The listing builds one solid part. Answer for the finished solid, in the listing's coordinates (mm). A direction names the side the tool comes from. Round coordinates to 2 decimals unless told otherwise and drop trailing zeros. Loops run counter-clockwise (first coordinate to the right, second up) from the corner with the lowest first, then second, coordinate; pieces in that order, holes last. Notation, with made-up numbers: (-19, -4.5) -> (4, -4.5) arc R12 ccw to (4, 2.5) -> close; hole circle Ø2 at (-19.75, 9). An arc over 180 degrees is marked (long way). Write each question's results on one line, items separated by ' | '. Start each with the question number.
(1) Determine the mould class of faces 1 (the face through (10, -8, -3)), 2 (the face through (4.93, 3.377, 3.849)), 3 (the face through (1.6, -11.8, -4)) for opening direction Z: released by +Z, released by -Z, zero draft, split by the parting line, or undercut.
(2) The part is cut by section C-C (y = 0). Determine the outline of the cut face in (x, z), plus the area to 3 significant figures.
(3) Flat-ended cylindrical pins translate along their axes: pin 1 (4 mm diameter, centred on x = 3.5, y = -4, fed in from +Z); pin 2 (2 mm diameter, centred on x = 0.5, z = -0.5, fed in from +Y); pin 3 (1.6 mm diameter, centred on x = 8.5, y = -12.5, fed in from +Z); pin 4 (6.5 mm diameter, centred on y = 0, z = 0, fed in from +X). Find the tip coordinate at first contact, or state that the pin passes through.
(4) The part is cut by section A-A (y = -10.75). Determine the outline of the cut face in (x, z), plus the area to 3 significant figures.
(5) Straight lines are drawn through the part: probe 1 along Z at (x, y) = (7.5, 0); probe 2 along X at (y, z) = (-9.75, 2); probe 3 along Z at (x, y) = (8.25, -17). For each, find the intervals that lie inside material, in ascending order.
(6) For faces 4 (the face through (8, -12, 2)), 5 (the face through (9, -11, -1.5)), 6 (the face through (1.6, -11.6, 4)), determine the directions among +Z, -Z, +X, -X, +Y, -Y from which every point of the face is accessible in a straight line to the end or side of a thin tool.
(7) The part is cut by section D-D (x = 4). Determine the outline of the cut face in (y, z).
(8) The part is cut by section B-B (z = 0). Determine the outline of the cut face in (x, y).
Autodesk Inventor part; units mm, degrees
ref_plane "YZ Plane" through (0, 0, 0) normal (1, 0, 0) x (0, 1, 0)
ref_plane "XZ Plane" through (0, 0, 0) normal (0, 1, 0) x (-1, 0, 0)
ref_plane "XY Plane" through (0, 0, 0) normal (0, 0, 1) x (1, 0, 0)
sketch "Sketch1" plane through (0, 0, 0) normal (1, 0, 0) x (0, 1, 0)
  arc A0 (2, 3.4641) -> (2, -3.4641) centre (0, 0) ccw
  arc A1 (2, 3.4641) -> (3, 5.1962) centre (2.5, 4.3301) ccw
  arc A2 (3, -5.1962) -> (2, -3.4641) centre (2.5, -4.3301) ccw
  line L0 (-4.4721, 4) -> (-19, 4)
  line L1 (-19, 4) -> (-19, -4)
  line L2 (-19, -4) -> (-4.4721, -4)
  arc A3 (3, 5.1962) -> (-4.4721, 4) centre (0, 0) ccw
  arc A4 (-4.4721, -4) -> (3, -5.1962) centre (0, 0) ccw
  point P0 (-6, 0)
  point P1 (-19, 0)
  dimension "d0" = 8
  dimension "d2" = 2.5
  dimension "d3" = 8
  dimension "d6" = 19
  dimension "d7" = 6
  dimension "d8" = 6
extrude "Extrusion1" add sketch "Sketch1" along normal blind 10
sketch "Sketch2" plane through (0, -19, 4) normal (0, 0, 1) x (1, 0, 0)
  line L0 (2, 12) -> (8, 12)
  line L1 (8, 12) -> (8, 2)
  line L2 (8, 2) -> (2, 2)
  line L3 (2, 2) -> (2, 12)
  line L4 (0, 0) -> (10, 0)
  line L5 (10, 14.5279) -> (10, 0)
  point P0 (0, 19)
  dimension "d11" = 2
  dimension "d12" = 6
  dimension "d13" = 10
  dimension "d14" = 2
extrude "Extrusion2" cut sketch "Sketch2" against normal blind 10
sketch "Sketch3" plane through (0, 0, 0) normal (-1, 0, 0) x (0, 0, 1)
  line L0 (-1.5, -7) -> (1.5, -7)
  line L1 (1.5, -7) -> (1.5, -15)
  line L2 (1.5, -15) -> (-1.5, -15)
  line L3 (-1.5, -15) -> (-1.5, -7)
  line L4 (4, -7) -> (-4, -7)
  line L5 (4, -17) -> (-4, -17)
  line L6 (4, -4.4721) -> (4, -19)
  point P0 (0, 0)
  point P1 (0, -7)
  point P2 (0, -7)
  dimension "d17" = 3
  dimension "d18" = 2
  dimension "d19" = 2.5
extrude "Extrusion3" cut sketch "Sketch3" against normal blind 10
properties part number "Thread_Clip"
Checked values:
1) face 1: zero draft | face 2: undercut | face 3: released by -Z
2) outline: (0, -6) -> (10, -6) -> (10, -4) -> (0, -4) -> close; (0, 4) -> (10, 4) -> (10, 6) -> (0, 6) -> close | area: 40.0 mm2
3) pin 1: stops at z = 5.66 | pin 2: stops at y = -3.71 | pin 3: stops at z = 4 | pin 4: passes through
4) outline: (0, -4) -> (2, -4) -> (2, -1.5) -> (0, -1.5) -> close; (0, 1.5) -> (2, 1.5) -> (2, 4) -> (0, 4) -> close; (8, -4) -> (10, -4) -> (10, -1.5) -> (8, -1.5) -> close; (8, 1.5) -> (10, 1.5) -> (10, 4) -> (8, 4) -> close | area: 20.0 mm2
5) probe 1: z = -6 to -4, 4 to 6 | probe 2: x = 0 to 2, 8 to 10 | probe 3: z = -4 to 4
6) face 4: +Z, -Z | face 5: +X, -X | face 6: +Z, +X, -X, -Y
7) outline: (-19, -4) -> (-17, -4) -> (-17, 4) -> (-19, 4) -> close; (-7, -4) -> (-4.47, -4) arc R6 ccw to (3, -5.2) arc R1 ccw to (2, -3.46) arc R4 cw (long way) to (2, 3.46) arc R1 ccw to (3, 5.2) arc R6 ccw to (-4.47, 4) -> (-7, 4) -> close
8) outline: (0, -19) -> (10, -19) -> (10, -15) -> (8, -15) -> (8, -17) -> (2, -17) -> (2, -15) -> (0, -15) -> close; (0, -7) -> (10, -7) -> (10, -4) -> (0, -4) -> close
